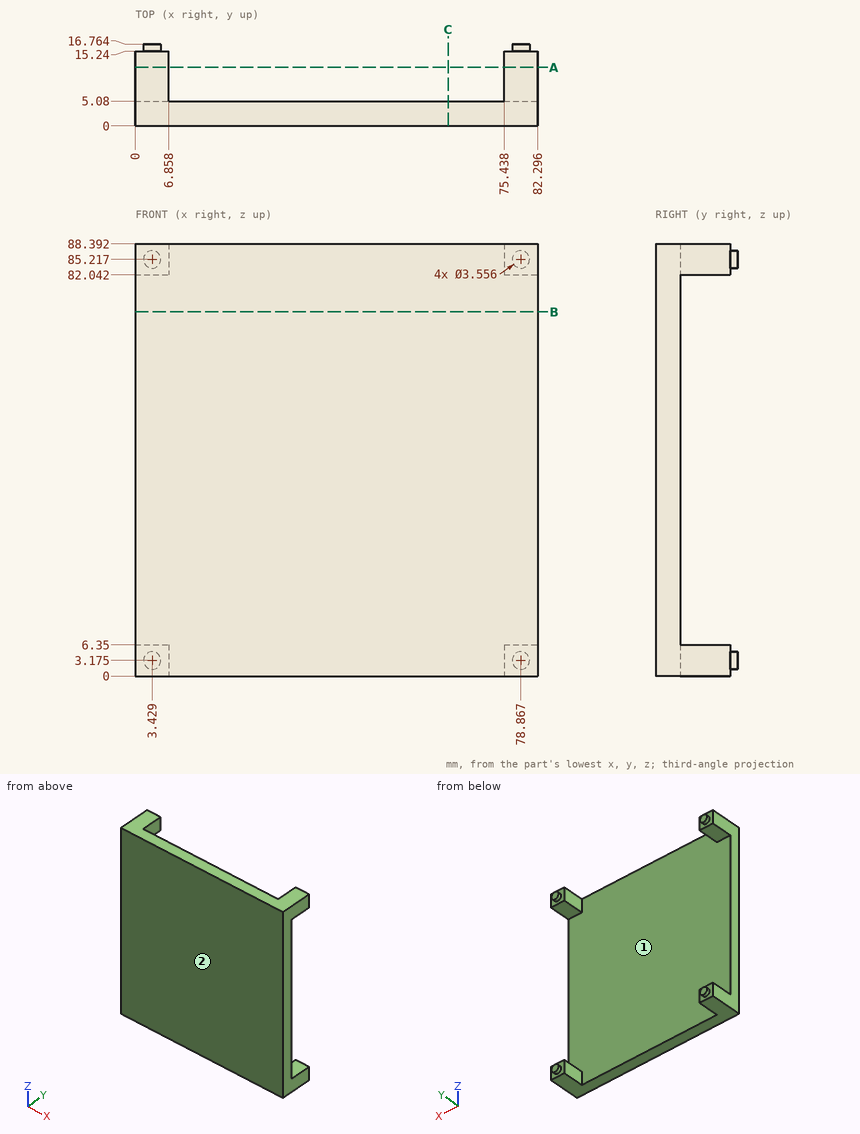
Geometry: see drawing. Coordinates: mm, zero at the bounding-box minimum. Give positions to 0.01 mm unless a question says otherwise; leave off trailing zeros. Order: outer loops, then holes, each group sorted by start corner. A loop starts at its lowest first (then second) coordinate and runs counter-clockwise, first axis right, second up. Notation, with made-up numbers: (59.5, 81) -> (71.5, 81) arc R18 cw to (71.5, 109) -> close; hole circle Ø11 at (89.25, 49). An arc over 180 degrees is marked (long way). Write item = value, one per line.
Q1. Pin query (flat end, axial travel): pin 1 (2 mm diameter, centred on x = 56, z = 23, fed in from -Y); pin 2 (10 mm diameter, centred on x = 18, y = 13, fed in from +Z); pin 3 (5 mm diameter, centred on x = 16, z = 33, fed in from +Y). Return the tip coordinate at first contact, or that it passes through.
Data:
pin_1 = 0
pin_2 = through
pin_3 = 5.08
Q2. Cut plane A-A, the plane y = 12. Output: boundary loops of the cut face in (x, z).
Data:
outline = (0, 0) -> (6.86, 0) -> (6.86, 6.35) -> (0, 6.35) -> close; (0, 82.04) -> (6.86, 82.04) -> (6.86, 88.39) -> (0, 88.39) -> close; (75.44, 0) -> (82.3, 0) -> (82.3, 6.35) -> (75.44, 6.35) -> close; (75.44, 82.04) -> (82.3, 82.04) -> (82.3, 88.39) -> (75.44, 88.39) -> close
Q3. Material intervals for line 1 (Y direction, x = 19.5, z = 48); line 2 (Z direction, x = 78.5, y = 14.75), sorted ascending. Write a range as from..to.
Data:
line_1 = 0..5.08
line_2 = 0..6.35, 82.04..88.39
Q4. Cut plane C-C, the plane x = 64. Output: boundary loops of the cut face in (y, z).
Data:
outline = (0, 0) -> (5.08, 0) -> (5.08, 88.39) -> (0, 88.39) -> close
Q5. Cut plane B-B, the plane z = 74.5. Output: boundary loops of the cut face in (x, y).
Data:
outline = (0, 0) -> (82.3, 0) -> (82.3, 5.08) -> (0, 5.08) -> close
Q6. Pull-direction query (Z, two-part tool) for the marked faces 1 and 2; classes: released by +Z, released by -Z, zero draft, split by the parting line, or undercut.
Data:
face_1 = undercut
face_2 = zero draft
